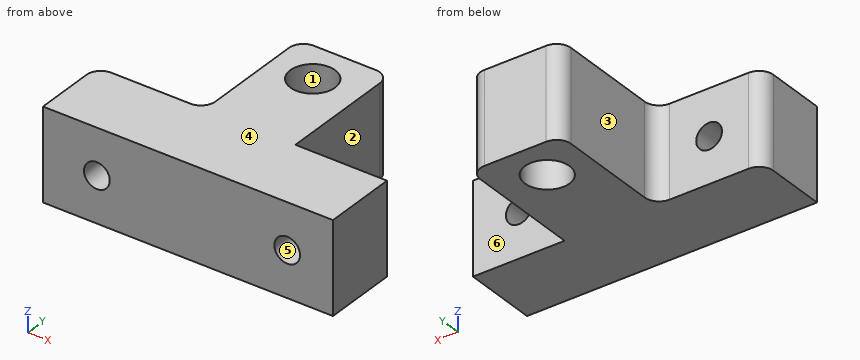
Autodesk Inventor part; units mm, degrees
ref_plane "FRONT" through (0, 0, 0) normal (0, 0, 1) x (1, 0, 0)
ref_plane "TOP" through (0, 0, 0) normal (0, 1, 0) x (-1, 0, 0)
ref_plane "RIGHT" through (0, 0, 0) normal (1, 0, 0) x (0, 1, 0)
ref_plane "FRONT" through (0, 0, 0) normal (0, 0, 1) x (1, 0, 0)
ref_plane "TOP" through (0, 0, 0) normal (0, 1, 0) x (-1, 0, 0)
ref_plane "RIGHT" through (0, 0, 0) normal (1, 0, 0) x (0, 1, 0)
ref_plane "Work Plane6" through (36, -22.5, -6.35) normal (0, 0, -1) x (-1, 0, 0)
sketch "Sketch1" plane through (36, -22.5, -6.35) normal (0, 0, -1) x (-1, 0, 0)
  line L0 (56.9176, 0) -> (29.4132, 0)
  line L1 (56.9176, 0) -> (29.4132, 0)
  line L2 (29.4132, 0) -> (29.4132, 32.1053)
  line L3 (41.9794, 32.1053) -> (41.9794, 16.7597)
  line L4 (29.4132, 32.1053) -> (41.9794, 32.1053)
  line L5 (41.9794, 16.7597) -> (56.9176, 16.7597)
  line L6 (56.9176, 16.7597) -> (56.9176, 0)
  point P0 (36, 22.5)
  point P1 (0, 0)
extrude "Extrusion1" add sketch "Sketch1" along normal blind 12.7
ref_plane "Work Plane5" through (36, -22.5, -19.05) normal (0, 0, -1) x (-1, 0, 0)
sketch "Sketch2" plane through (36, -22.5, -19.05) normal (0, 0, -1) x (-1, 0, 0)
  circle A0 centre (36, 22.5) radius 3.1
  dimension "d2" = 6.2
extrude "Extrusion2" cut sketch "Sketch2" against normal through all
ref_plane "Work Plane8" through (6.5868, -22.5, -6.35) normal (1, 0, 0) x (0, 0, -1)
sketch "Sketch3" plane through (6.5868, -22.5, -6.35) normal (1, 0, 0) x (0, 0, -1)
  line L0 (0, 32.1053) -> (0, 0)
  line L1 (0, 13.4651) -> (12.7, 13.4651)
  line L2 (12.7, 13.4651) -> (12.7, 0)
  line L3 (12.7, 0) -> (0, 0)
  line L4 (0, 0) -> (0, 13.4651)
  point P0 (-6.35, 22.5)
  point P1 (0, 26.9303)
extrude "Extrusion3" add sketch "Sketch3" along normal blind 12.7
sketch "Sketch4" plane through (36, -22.5, -19.05) normal (0, 0, -1) x (-1, 0, 0)
  circle A0 centre (36, 22.5) radius 3.1
  line L0 (29.4132, 32.1053) -> (29.4132, 13.4651)
  line L1 (56.9176, 0) -> (16.7132, 0)
  line L2 (56.9176, 0) -> (56.9176, 16.7597)
  line L3 (56.9176, 16.7597) -> (41.9794, 16.7597)
  line L4 (41.9794, 16.7597) -> (41.9794, 32.1053)
  line L5 (41.9794, 32.1053) -> (29.4132, 32.1053)
  line L6 (16.7132, 0) -> (16.7132, 13.4651)
  line L7 (16.7132, 10.2251) -> (56.9176, 10.2251)
  line L8 (56.9176, 0) -> (56.9176, 16.7597)
  line L9 (41.9794, 16.7597) -> (41.9794, 10.2251)
  line L10 (29.4132, 13.4651) -> (29.4132, 10.2251)
  line L11 (29.4132, 13.4651) -> (16.7132, 13.4651)
  line L12 (16.7132, 13.4651) -> (16.7132, 10.2251)
  line L13 (41.9794, 16.7597) -> (56.9176, 16.7597)
  line L14 (56.9176, 16.7597) -> (56.9176, 10.2251)
  line L15 (29.4132, 13.4651) -> (16.7132, 13.4651)
  line L16 (16.7132, 13.4651) -> (16.7132, 10.2251)
  line L17 (16.7132, 10.2251) -> (29.4132, 10.2251)
  line L18 (29.4132, 10.2251) -> (29.4132, 13.4651)
  line L19 (41.9794, 16.7597) -> (56.9176, 16.7597)
  line L20 (56.9176, 16.7597) -> (56.9176, 10.2251)
  line L21 (56.9176, 10.2251) -> (41.9794, 10.2251)
  line L22 (41.9794, 10.2251) -> (41.9794, 16.7597)
  line L23 (29.4132, 13.4651) -> (16.7132, 13.4651)
  line L24 (16.7132, 0) -> (16.7132, 13.4651)
extrude "Extrusion4" cut sketch "Sketch4" against normal through all contours L10 L7 L6 L11 | L3 L2 L7 L9
sketch "Sketch5" plane through (36, -22.5, -19.05) normal (0, 0, -1) x (-1, 0, 0)
  line L0 (56.9176, 0) -> (16.7132, 0)
  line L1 (56.9176, 0) -> (56.9176, 10.2251)
  line L2 (56.9176, 10.2251) -> (41.9794, 10.2251)
  line L3 (41.9794, 10.2251) -> (41.9794, 32.1053)
  line L4 (41.9794, 32.1053) -> (29.4132, 32.1053)
  line L5 (29.4132, 32.1053) -> (29.4132, 10.2251)
  circle A0 centre (36, 22.5) radius 3.1
  line L6 (29.4132, 32.1053) -> (29.4132, 10.2251)
  line L7 (29.4132, 28.1591) -> (41.9794, 28.1591)
  line L8 (41.9794, 28.1591) -> (41.9794, 32.1053)
  line L9 (41.9794, 32.1053) -> (29.4132, 32.1053)
  line L10 (29.4132, 32.1053) -> (29.4132, 28.1591)
  line L11 (29.4132, 10.2251) -> (16.7132, 10.2251)
  line L12 (16.7132, 0) -> (16.7132, 10.2251)
extrude "Extrusion5" cut sketch "Sketch5" against normal through all contours L7 L5 L4 L3
fillet "Fillet4" radius 2 4 edges at (-5.9794, 5.6591, -12.7) (-5.9794, -12.2749, -12.7) (6.5868, 5.6591, -12.7) (-20.9176, -12.2749, -12.7)
ref_plane "Work Plane9" through (8.5868, -12.2749, -19.05) normal (0, 1, 0) x (1, 0, 0)
sketch "Sketch6" plane through (8.5868, -12.2749, -19.05) normal (0, 1, 0) x (1, 0, 0)
  line L0 (-2, 0) -> (10.7, 0)
  line L1 (10.7, -12.7) -> (-2, -12.7)
  line L2 (8.7, -6.35) -> (0, -6.35) construction
  line L3 (0, -12.7) -> (0, 0) construction
  line L4 (-29.5044, 0) -> (10.7, 0) construction
  line L5 (4.35, 0) -> (4.35, -12.7) construction
  line L6 (-29.5044, -12.7) -> (10.7, -12.7) construction
  circle A0 centre (4.35, -6.35) radius 1.7859
  line L7 (10.7, 0) -> (10.7, -12.7)
  line L8 (-2, 0) -> (-2, -12.7)
  point P0 (-8.5868, -19.05)
  point P1 (8.7, -12.7)
  point P2 (8.7, 0)
  dimension "d18" = 3.5719
extrude "Extrusion6" cut sketch "Sketch6" against normal through all contours A0
sketch "Sketch7" plane through (-18.9176, -12.2749, -19.05) normal (0, 1, 0) x (1, 0, 0)
  line L0 (0, -12.7) -> (0, 0)
  line L1 (10.9382, -12.7) -> (0, -12.7)
  line L2 (10.9382, 0) -> (10.9382, -12.7)
  line L3 (0, 0) -> (10.9382, 0)
  line L4 (5.4691, -12.7) -> (5.4691, 0) construction
  line L5 (-2, 0) -> (38.2044, 0) construction
  line L6 (10.9382, 0) -> (10.9382, -12.7) construction
  line L7 (10.9382, -6.35) -> (0, -6.35) construction
  circle A0 centre (5.4691, -6.35) radius 1.7859
  point P0 (18.9176, -19.05)
  point P1 (25.5044, 0)
  dimension "d21" = 3.5719
extrude "Extrusion7" cut sketch "Sketch7" against normal through all contours A0
properties part number "other side roller axle holder"
Can you work these out from the model? Positions are in its coordinate system, mm. Face numbers are marked on the shaded views. A direction names the side the tool comes from. Round coordinates to 2 decimals unless told otherwise and drop trailing zeros. Order: outer loops, then holes, each group sorted by start corner. A loop starts at its lowest first (then second) coordinate and runs counter-clockwise, first axis right, second up. Notation, with made-up numbers: M 53,7.5 L 101,7.5 A32 cw 101,34.5 Z; hole C -12,46 d9. An arc over 180 degrees is marked long. Use a Markdown table: item, result.
1) Imagine slicing it at D-D (z = -16.25). List the corners of the cut face in (x, y) for me.
Geometry says:
| item | result |
|---|---|
| outline | M -20.92,-22.5 L 19.29,-22.5 L 19.29,-12.27 L 6.59,-12.27 L 6.59,3.66 A2 ccw 4.59,5.66 L -3.98,5.66 A2 ccw -5.98,3.66 L -5.98,-10.27 A2 cw -7.98,-12.27 L -18.92,-12.27 A2 ccw -20.92,-14.27 Z; hole C 0,0 d6.2 |
2) I'm going to push flat-ended pins straight in: P1, Ø3, axis at y = -6.5, z = -12.5, coming from the +X side; P2, Ø10, axis at x = -6.5, y = 0, coming from the -Z side; P3, Ø4, axis at x = 13.5, z = -13.5, coming from the +Y side. Where does each tip first touch, or does it pass through?
Geometry says:
| item | result |
|---|---|
| P1 | stops at x = 6.59 |
| P2 | stops at z = -19.05 |
| P3 | stops at y = -12.27 |
3) If I drill on line 1 along X through (y, z) = (-19.5, -12.7); line 2 along Y through (x, z) = (0, -11); line 3 along Y through (x, z) = (15, -10.75), over which ranges is the centre line in solid material (lowest first)?
Geometry says:
| item | result |
|---|---|
| line 1 | x = -20.92 to -15.23, -11.66 to 11.15, 14.72 to 19.29 |
| line 2 | y = -22.5 to -3.1, 3.1 to 5.66 |
| line 3 | y = -22.5 to -12.27 |
4) Imagine slicing it at B-B (z = -12.7). List the corners of the cut face in (x, y) for me.
Geometry says:
| item | result |
|---|---|
| outline | M -20.92,-22.5 L -15.23,-22.5 L -15.23,-12.27 L -18.92,-12.27 A2 ccw -20.92,-14.27 Z; M -11.66,-22.5 L 11.15,-22.5 L 11.15,-12.27 L 6.59,-12.27 L 6.59,3.66 A2 ccw 4.59,5.66 L -3.98,5.66 A2 ccw -5.98,3.66 L -5.98,-10.27 A2 cw -7.98,-12.27 L -11.66,-12.27 Z; M 14.72,-22.5 L 19.29,-22.5 L 19.29,-12.27 L 14.72,-12.27 Z; hole C 0,0 d6.2 |
5) If we mould it in two halves opening along Z, with no side actions, what happens to the marked faces 4, 5 and 6? For each: +Z half, -Z half, draft (parallel to the pull), parting line (faces both ways), or undercut.
Geometry says:
| item | result |
|---|---|
| face 4 | +Z half |
| face 5 | undercut |
| face 6 | draft |
6) On a 3-axis mill with a long thin cutter (end or side, diameter ignored), from which of +Z, -Z, +X, -X, +Y, -Y can I reach the whole of each face in a straight line? I mean the marked faces 1, 2 and 3. Say none if no direction works.
Geometry says:
| item | result |
|---|---|
| face 1 | +Z, -Z |
| face 2 | +Z, -Z, +X, +Y |
| face 3 | +Z, -Z, -X, +Y |
7) Imagine slicing it at A-A (y = 0). List the corners of the cut face in (x, z) for me, then the cut area to 3 significant figures.
Geometry says:
| item | result |
|---|---|
| outline | M -5.98,-19.05 L -3.1,-19.05 L -3.1,-6.35 L -5.98,-6.35 Z; M 3.1,-19.05 L 6.59,-19.05 L 6.59,-6.35 L 3.1,-6.35 Z |
| area | 80.9 mm² |
8) Imagine slicing it at C-C (x = 0). List the corners of the cut face in (y, z) for me.
Geometry says:
| item | result |
|---|---|
| outline | M -22.5,-19.05 L -3.1,-19.05 L -3.1,-6.35 L -22.5,-6.35 Z; M 3.1,-19.05 L 5.66,-19.05 L 5.66,-6.35 L 3.1,-6.35 Z |
